Read the model definition and answer for the solid it produces. Units are mm, in the model's axes. Give positions to 0.01 mm unless a question says otherwise; leave off trailing zeros. Write each loop counter-clockwise with the first axis right and the second up, starting at its lowest first coordinate (ties: lowest second). Pieces come first, ordered by that corner, then holes. Notation, with made-up numbers: (-24.5, 72.25) -> (29.5, 72.25) arc R12 ccw to (29.5, 94.25) -> close; hole circle Ø3 at (-27.75, 74). An arc over 180 degrees is marked (long way). Answer as CSV lines item,"result". Start each with the question number.
1. The part is cut by section A-A, the plane x = 0. Determine the outline of the cut face in (y, z), and give its area (3 significant figures).
2. The part is cut by section C-C, the plane z = 32. Determine the outline of the cut face in (x, y), and give its area (3 significant figures).
3. For a pull along Y with two mould halves and no side action, classify faces 1 (the cylindrical face through (-10.154, -77.336, 90.145)), 2 (the cylindrical face through (-58.23, 53.39, 87.66)), 3 (the flat face through (58.1, -52.3, 0)) as pulls with the +Y half, pulls with the -Y half, needs draft (parallel to the pull), parting line crosses it, or undercut.
4. Given pin 1 (2 mm diameter, centred on x = 62.5, z = 116, fed in from -Y); pin 2 (12 mm diameter, centred on x = -13.5, z = 105, fed in from +Y); pin 3 (2 mm diameter, centred on y = -53.5, z = 138.5, fed in from +X), each flat-ended and moving along its own axis, determine where each tip first touches the part or whether it passes through.
5. Find the intervals of material crossed by line 1 (Y direction, x = 0, z = 38); line 2 (X direction, y = 39.5, z = 170); line 3 (X direction, y = 55, z = 92.5), in increasing order.
from build123d import *

# Parameters (mm, degrees)
F0_R     = 79
F1_DEPTH = 177.8
F2_T     = -1
F3_DEPTH = 1.001
F4_R     = 2
F5_DEPTH = 110


with BuildPart() as f1:
    # F0 (on Top) → F1 (new body)
    with BuildSketch(Plane.XY):
        Circle(F0_R)
    extrude(amount=F1_DEPTH)

    # F2
    f2_openings = [f1.faces().sort_by_distance(p)[0] for p in [
        (0, 0, 177.8),
    ]]
    offset(amount=F2_T, openings=f2_openings)

    # F3 (cut, through all): a face of the model
    f3_faces = [f1.faces().sort_by_distance(p)[0] for p in [
        (0, 0, 1),
    ]]
    extrude(f3_faces, amount=-F3_DEPTH, mode=Mode.SUBTRACT)


with BuildPart() as f5:
    # F4 (on Top) → F5 (new body)
    with BuildSketch(Plane.XY):
        with Locations((-59.2270195484, 59.6657395363)):
            Circle(F4_R)
    extrude(amount=F5_DEPTH)


solid = f1.part
Results found:
1,outline,"(-79, 0) -> (-78, 0) -> (-78, 177.8) -> (-79, 177.8) -> close; (78, 0) -> (79, 0) -> (79, 177.8) -> (78, 177.8) -> close"
1,area,"356 mm²"
2,outline,"circle Ø158 at (0, 0); hole circle Ø156 at (0, 0)"
2,area,"493 mm²"
3,face 1,"undercut"
3,face 2,"parting line crosses it"
3,face 3,"needs draft"
4,pin 1,"stops at y = -49.59"
4,pin 2,"stops at y = 78.64"
4,pin 3,"stops at x = 59.03"
5,line 1,"y = -79 to -78, 78 to 79"
5,line 2,"x = -68.42 to -67.26, 67.26 to 68.42"
5,line 3,"x = -56.71 to -55.31, 55.31 to 56.71"
